Can you work these out from the model? Positions are in its coordinate system, mm. Round coordinates to 2 decimals unless told otherwise and drop trailing zeros. Order: outer loops, then holes, each group sorted by start corner. A loop starts at its lowest first (then second) coordinate and runs counter-clockwise, first axis right, second up. Notation, with made-up numbers: (44, -12) -> (64, -12) arc R27 cw to (64, 20) -> close; hole circle Ø2 at (-12.75, 27.5). An arc over 180 degrees is marked (long way). Use a Markdown table: item, result. Add a question column.
Q1. I'm going to push flat-ended pins straight in: pin 1 Ø8 at (y, z) = (82.5, 50.5) entering from +X; pin 2 Ø5.5 at (x, y) = (2.5, 80) entering from +Z; pin 3 Ø1 at (x, z) = (8, 25) entering from +Y; pin 4 Ø1.5 at (x, y) = (4.5, -85) entering from -Z. Where does each tip first touch, or does it pass through?
Q2. I need wall thicknesses on line 1 along Y through (x, z) = (4, -14.5); line 2 along X through (y, z) = (77.5, -44.5). Which ranges of each line are inside material? Lowest first, please. Write a range as [from, to].
Q3. If we section it at B-B on y = -82.5: List the corners of the cut face in (x, z) for me.
Q4. If we section it at A-A on z = 50.5: List the corners of the cut face in (x, y) for me, plus the area to 3 significant figures.
Q5. If we section it at D-D on x = 26: List the corners of the cut face in (y, z) for me.
Q6. If we section it at C-C on z = 12.5: List the corners of the cut face in (x, y) for me.
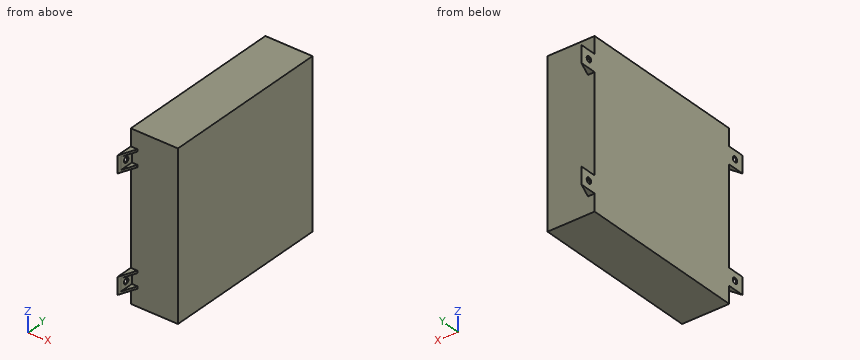
```python
from build123d import *

# Parameters (mm, degrees)
SKETCH_1_W            = 146
SKETCH_1_H            = 152
EXTRUDE_1_DEPTH       = 42
EXTRUDE_2_DEPTH       = 15
MIRROR_2_COPY_1_DEPTH = 15
CUT_EXTRUDE_START     = -2
CUT_EXTRUDE_1_DEPTH   = 11
MIRROR_START          = -2
MIRROR_4_COPY_1_DEPTH = 11
SKETCH_4_R            = 2.5
CUT_EXTRUDE_2_DEPTH   = 11


with BuildPart() as part:
    # 草图1 → 凸台-拉伸1 (new body)
    with BuildSketch(Plane(origin=(0, 0, 0), x_dir=(0, 0, -1), z_dir=(1, 0, 0))):
        Rectangle(SKETCH_1_W, SKETCH_1_H)
    extrude(amount=EXTRUDE_1_DEPTH)

    # 草图2 → 凸台-拉伸2 (add)
    with BuildSketch(Plane.XY.offset(58)):
        Polygon((0, -76), (0, -91), (6, -76), align=None)
    extrude_2 = extrude(amount=-EXTRUDE_2_DEPTH)

    # 镜向1: 凸台-拉伸2 across plane
    add(extrude_2.mirror(Plane(origin=(0, 0, 0), x_dir=(0, 0, 1), z_dir=(0, -1, 0))))

    # 镜向2: 凸台-拉伸2 across plane
    add(extrude_2.mirror(Plane(origin=(0, 0, 0), x_dir=(1, 0, 0), z_dir=(0, 0, -1))))

    # 镜向2 copy 1 sketch → 镜向2 copy 1 (add)
    with BuildSketch(Plane(origin=(0, 0, -58), x_dir=(1, 0, 0), z_dir=(0, 0, -1))):
        Polygon((0, -76), (0, -91), (6, -76), align=None)
    extrude(amount=-MIRROR_2_COPY_1_DEPTH)

    # 草图3 → 切除-拉伸1 (cut)
    with BuildSketch(Plane.XY.offset(58).offset(CUT_EXTRUDE_START)):
        Polygon((6, -76), (1, -88.5), (1, -76), align=None)
    cut_extrude_1 = extrude(amount=-CUT_EXTRUDE_1_DEPTH, mode=Mode.SUBTRACT)

    # 镜向3: 切除-拉伸1 across plane
    add(cut_extrude_1.mirror(Plane(origin=(0, 0, 0), x_dir=(1, 0, 0), z_dir=(0, 0, -1))), mode=Mode.SUBTRACT)

    # 镜向4: 切除-拉伸1 across plane
    add(cut_extrude_1.mirror(Plane(origin=(0, 0, 0), x_dir=(0, 0, 1), z_dir=(0, -1, 0))), mode=Mode.SUBTRACT)

    # 镜向4 copy 1 sketch → 镜向4 copy 1 (cut)
    with BuildSketch(Plane(origin=(0, 0, -58), x_dir=(1, 0, 0), z_dir=(0, 0, -1)).offset(MIRROR_START)):
        Polygon((6, -76), (1, -88.5), (1, -76), align=None)
    extrude(amount=-MIRROR_4_COPY_1_DEPTH, mode=Mode.SUBTRACT)

    # 草图4 → 切除-拉伸2 (cut)
    with BuildSketch(Plane(origin=(1, 0, 0), x_dir=(0, 0, -1), z_dir=(1, 0, 0))):
        with Locations((-50.5, -82.5)):
            Circle(SKETCH_4_R)
        with Locations((50.5, -82.5)):
            Circle(SKETCH_4_R)
        with Locations((-50.5, 82.5)):
            Circle(SKETCH_4_R)
        with Locations((50.5, 82.5)):
            Circle(SKETCH_4_R)
    extrude(amount=-CUT_EXTRUDE_2_DEPTH, mode=Mode.SUBTRACT)


solid = part.part
```
Answer below:
| question | item | result |
|---|---|---|
| 1 | pin 1 | x = 1 |
| 1 | pin 2 | z = 58 |
| 1 | pin 3 | y = 76 |
| 1 | pin 4 | through |
| 2 | line 1 | [-76, 76] |
| 2 | line 2 | [0, 5.4] |
| 3 | outline | (0, -58) -> (3.4, -58) -> (3.4, -56) -> (1, -56) -> (1, -53) -> (0, -53) -> close; (0, -48) -> (1, -48) -> (1, -45) -> (3.4, -45) -> (3.4, -43) -> (0, -43) -> close; (0, 43) -> (3.4, 43) -> (3.4, 45) -> (1, 45) -> (1, 48) -> (0, 48) -> close; (0, 53) -> (1, 53) -> (1, 56) -> (3.4, 56) -> (3.4, 58) -> (0, 58) -> close |
| 4 | outline | (0, -91) -> (1, -88.5) -> (1, -85) -> (0, -85) -> close; (0, -80) -> (1, -80) -> (1, -76) -> (42, -76) -> (42, 76) -> (1, 76) -> (1, 80) -> (0, 80) -> close; (0, 85) -> (1, 85) -> (1, 88.5) -> (0, 91) -> close |
| 4 | area | 6,400 mm² |
| 5 | outline | (-76, -73) -> (76, -73) -> (76, 73) -> (-76, 73) -> close |
| 6 | outline | (0, -76) -> (42, -76) -> (42, 76) -> (0, 76) -> close |
